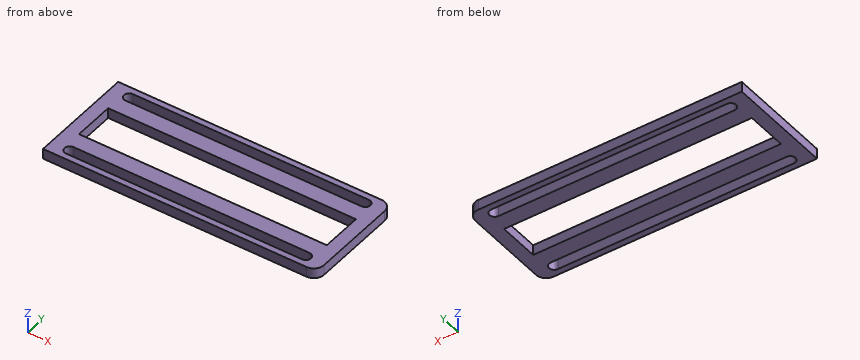
```python
from build123d import *

# Parameters (mm, degrees)
SKETCH003_W   = 80
SKETCH003_H   = 31
SKETCH003_W_2 = 72.408426
SKETCH003_H_2 = 12
EXTRUDE_DEPTH = 3
FILLET_R      = 3


with BuildPart() as part:
    # Sketch003 → Extrude (new body)
    with BuildSketch(Plane.XY):
        Rectangle(SKETCH003_W, SKETCH003_H)
        Rectangle(SKETCH003_W_2, SKETCH003_H_2, mode=Mode.SUBTRACT)
        with BuildLine():
            ThreePointArc((-34.5, 13.75), (-36, 12.25), (-34.5, 10.75))
            Line((-34.5, 10.75), (34.5, 10.75))
            ThreePointArc((34.5, 10.75), (36, 12.25), (34.5, 13.75))
            Line((-34.5, 13.75), (34.5, 13.75))
        make_face(mode=Mode.SUBTRACT)
        with BuildLine():
            ThreePointArc((-34.5, -10.75), (-36, -12.25), (-34.5, -13.75))
            Line((-34.5, -13.75), (34.5, -13.75))
            ThreePointArc((34.5, -13.75), (36, -12.25), (34.5, -10.75))
            Line((-34.5, -10.75), (34.5, -10.75))
        make_face(mode=Mode.SUBTRACT)
    extrude(amount=EXTRUDE_DEPTH)

    # Fillet
    fillet_edges = [part.edges().sort_by_distance(p)[0] for p in [
        (40, 15.5, 1.5),
        (40, -15.5, 1.5),
    ]]
    fillet(fillet_edges, radius=FILLET_R)


solid = part.part
```
The model under review builds one solid part; all positions refer to its coordinate system, in mm. Round coordinates to 2 decimals unless told otherwise and drop trailing zeros. Write each loop counter-clockwise with the first axis right and the second up, starting at its lowest first coordinate (ties: lowest second). Pieces come first, ordered by that corner, then holes.
(1) We need section C-C on z = 2. Give the boundary of the cut face in (x, y).
(2) We need section A-A on y = 4.5. Give the boundary of the cut face in (x, z).
(3) We need section B-B on x = 28. Give the boundary of the cut face in (y, z), and give its area (3 significant figures).
(4) Wall thickness on L1, parallel to Y at x = 6, z = 2.2; L2, parallel to X at y = 0, z = 1.45; L3, parallel to X at y = -13, z = 2.1: over which ranges is each line inside the solid? List them lowest first.
Findings below:
1. outline: (-40, -15.5) - (37, -15.5) arc R3 ccw to (40, -12.5) - (40, 12.5) arc R3 ccw to (37, 15.5) - (-40, 15.5) - close; hole (-36.2, -6) - (36.2, -6) - (36.2, 6) - (-36.2, 6) - close; hole (-34.5, -13.75) - (34.5, -13.75) arc R1.5 ccw to (34.5, -10.75) - (-34.5, -10.75) arc R1.5 ccw to start; hole (-34.5, 10.75) - (34.5, 10.75) arc R1.5 ccw to (34.5, 13.75) - (-34.5, 13.75) arc R1.5 ccw to start
2. outline: (-40, 0) - (-36.2, 0) - (-36.2, 3) - (-40, 3) - close; (36.2, 0) - (40, 0) - (40, 3) - (36.2, 3) - close
3. outline: (-15.5, 0) - (-13.75, 0) - (-13.75, 3) - (-15.5, 3) - close; (-10.75, 0) - (-6, 0) - (-6, 3) - (-10.75, 3) - close; (6, 0) - (10.75, 0) - (10.75, 3) - (6, 3) - close; (13.75, 0) - (15.5, 0) - (15.5, 3) - (13.75, 3) - close
3. area: 39.0 mm2
4. L1: y = -15.5 to -13.75, -10.75 to -6, 6 to 10.75, 13.75 to 15.5
4. L2: x = -40 to -36.2, 36.2 to 40
4. L3: x = -40 to -35.8, 35.8 to 39.96
